Work out the finished part from the listing and answer in its coordinate system (mm). Face numbers are marked on the shaded views. A direction names the side the tool comes from. Give positions to 0.01 mm unless a question says otherwise; leave off trailing zeros. Loops run counter-clockwise (first coordinate to the right, second up) from the corner with the lowest first, then second, coordinate; pieces in that order, holes last. Notation, with made-up numbers: M 83,10 L 114,10 A20 cw 114,25 Z; hole C -2.5,-19 d6. An arc over 180 degrees is marked long. Use a Markdown table: item, result.
```python
from build123d import *

# Parameters (mm, degrees)
BOSS_EXTRUDE1_DEPTH = 1.8
SKETCH2_R           = 3.25
SKETCH2_R_2         = 2.5
BOSS_EXTRUDE3_DEPTH = 0.2
SKETCH4_R           = 3.25
SKETCH4_R_2         = 2
BOSS_EXTRUDE4_DEPTH = 3
CUT_EXTRUDE1_REACH  = 4
SKETCH5_R           = 1.5
CUT_EXTRUDE2_REACH  = 6.8
SKETCH6_R           = 0.5


with BuildPart() as part:
    # Sketch1 → Boss-Extrude1 (new body)
    with BuildSketch(Plane.XY):
        with BuildLine():
            Line((1.525163579, 2.869908719), (15.645, 1.543202838))
            ThreePointArc((15.645, 1.543202838), (17.05, 0), (15.645, -1.543202838))
            Line((15.645, -1.543202838), (1.525163579, -2.869908719))
            ThreePointArc((1.525163579, -2.869908719), (0, -3.25), (-1.525163579, -2.869908719))
            Line((-1.525163579, -2.869908719), (-15.645, -1.543202838))
            ThreePointArc((-15.645, -1.543202838), (-17.05, 0), (-15.645, 1.543202838))
            Line((-15.645, 1.543202838), (-1.525163579, 2.869908719))
            ThreePointArc((-1.525163579, 2.869908719), (0, 3.25), (1.525163579, 2.869908719))
        make_face()
    extrude(amount=BOSS_EXTRUDE1_DEPTH)

    # Sketch2 → Boss-Extrude3 (add)
    with BuildSketch(Plane(origin=(0, 0, 0), x_dir=(-1, 0, 0), z_dir=(0, 0, -1))):
        Circle(SKETCH2_R)
        Circle(SKETCH2_R_2, mode=Mode.SUBTRACT)
    extrude(amount=BOSS_EXTRUDE3_DEPTH)

    # Sketch4 → Boss-Extrude4 (add)
    with BuildSketch(Plane.XY.offset(1.8)):
        Circle(SKETCH4_R)
        Circle(SKETCH4_R_2, mode=Mode.SUBTRACT)
    extrude(amount=BOSS_EXTRUDE4_DEPTH)

    # Sketch5 → Cut-Extrude1 (cut, up to next)
    with BuildSketch(Plane.XY.offset(1.8), mode=Mode.PRIVATE) as cut_extrude1_sk1:
        Circle(SKETCH5_R)
    cut_extrude1_tool1 = extrude(cut_extrude1_sk1.sketch, amount=-CUT_EXTRUDE1_REACH, mode=Mode.PRIVATE) & part.part
    add(cut_extrude1_tool1.solids().sort_by_distance((0, 0, 1.8))[0], mode=Mode.SUBTRACT)

    # Sketch6 → Cut-Extrude2 (cut, up to next)
    with BuildSketch(Plane(origin=(0, 0, 0), x_dir=(-1, 0, 0), z_dir=(0, 0, -1)), mode=Mode.PRIVATE) as cut_extrude2_sk1:
        with Locations((15.5, 0)):
            Circle(SKETCH6_R)
    cut_extrude2_tool1 = extrude(cut_extrude2_sk1.sketch, amount=-CUT_EXTRUDE2_REACH, mode=Mode.PRIVATE) & part.part
    add(cut_extrude2_tool1.solids().sort_by_distance((-15.5, 0, 0))[0], mode=Mode.SUBTRACT)
    # Sketch6 → Cut-Extrude2 (cut, up to next)
    with BuildSketch(Plane(origin=(0, 0, 0), x_dir=(-1, 0, 0), z_dir=(0, 0, -1)), mode=Mode.PRIVATE) as cut_extrude2_sk2:
        with Locations((13.3, 0)):
            Circle(SKETCH6_R)
    cut_extrude2_tool2 = extrude(cut_extrude2_sk2.sketch, amount=-CUT_EXTRUDE2_REACH, mode=Mode.PRIVATE) & part.part
    add(cut_extrude2_tool2.solids().sort_by_distance((-13.3, 0, 0))[0], mode=Mode.SUBTRACT)
    # Sketch6 → Cut-Extrude2 (cut, up to next)
    with BuildSketch(Plane(origin=(0, 0, 0), x_dir=(-1, 0, 0), z_dir=(0, 0, -1)), mode=Mode.PRIVATE) as cut_extrude2_sk3:
        with Locations((11.1, 0)):
            Circle(SKETCH6_R)
    cut_extrude2_tool3 = extrude(cut_extrude2_sk3.sketch, amount=-CUT_EXTRUDE2_REACH, mode=Mode.PRIVATE) & part.part
    add(cut_extrude2_tool3.solids().sort_by_distance((-11.1, 0, 0))[0], mode=Mode.SUBTRACT)
    # Sketch6 → Cut-Extrude2 (cut, up to next)
    with BuildSketch(Plane(origin=(0, 0, 0), x_dir=(-1, 0, 0), z_dir=(0, 0, -1)), mode=Mode.PRIVATE) as cut_extrude2_sk4:
        with Locations((8.9, 0)):
            Circle(SKETCH6_R)
    cut_extrude2_tool4 = extrude(cut_extrude2_sk4.sketch, amount=-CUT_EXTRUDE2_REACH, mode=Mode.PRIVATE) & part.part
    add(cut_extrude2_tool4.solids().sort_by_distance((-8.9, 0, 0))[0], mode=Mode.SUBTRACT)
    # Sketch6 → Cut-Extrude2 (cut, up to next)
    with BuildSketch(Plane(origin=(0, 0, 0), x_dir=(-1, 0, 0), z_dir=(0, 0, -1)), mode=Mode.PRIVATE) as cut_extrude2_sk5:
        with Locations((6.7, 0)):
            Circle(SKETCH6_R)
    cut_extrude2_tool5 = extrude(cut_extrude2_sk5.sketch, amount=-CUT_EXTRUDE2_REACH, mode=Mode.PRIVATE) & part.part
    add(cut_extrude2_tool5.solids().sort_by_distance((-6.7, 0, 0))[0], mode=Mode.SUBTRACT)
    # Sketch6 → Cut-Extrude2 (cut, up to next)
    with BuildSketch(Plane(origin=(0, 0, 0), x_dir=(-1, 0, 0), z_dir=(0, 0, -1)), mode=Mode.PRIVATE) as cut_extrude2_sk6:
        with Locations((4.5, 0)):
            Circle(SKETCH6_R)
    cut_extrude2_tool6 = extrude(cut_extrude2_sk6.sketch, amount=-CUT_EXTRUDE2_REACH, mode=Mode.PRIVATE) & part.part
    add(cut_extrude2_tool6.solids().sort_by_distance((-4.5, 0, 0))[0], mode=Mode.SUBTRACT)
    # Sketch6 → Cut-Extrude2 (cut, up to next)
    with BuildSketch(Plane(origin=(0, 0, 0), x_dir=(-1, 0, 0), z_dir=(0, 0, -1)), mode=Mode.PRIVATE) as cut_extrude2_sk7:
        with Locations((-4.5, 0)):
            Circle(SKETCH6_R)
    cut_extrude2_tool7 = extrude(cut_extrude2_sk7.sketch, amount=-CUT_EXTRUDE2_REACH, mode=Mode.PRIVATE) & part.part
    add(cut_extrude2_tool7.solids().sort_by_distance((4.5, 0, 0))[0], mode=Mode.SUBTRACT)
    # Sketch6 → Cut-Extrude2 (cut, up to next)
    with BuildSketch(Plane(origin=(0, 0, 0), x_dir=(-1, 0, 0), z_dir=(0, 0, -1)), mode=Mode.PRIVATE) as cut_extrude2_sk8:
        with Locations((-6.7, 0)):
            Circle(SKETCH6_R)
    cut_extrude2_tool8 = extrude(cut_extrude2_sk8.sketch, amount=-CUT_EXTRUDE2_REACH, mode=Mode.PRIVATE) & part.part
    add(cut_extrude2_tool8.solids().sort_by_distance((6.7, 0, 0))[0], mode=Mode.SUBTRACT)
    # Sketch6 → Cut-Extrude2 (cut, up to next)
    with BuildSketch(Plane(origin=(0, 0, 0), x_dir=(-1, 0, 0), z_dir=(0, 0, -1)), mode=Mode.PRIVATE) as cut_extrude2_sk9:
        with Locations((-8.9, 0)):
            Circle(SKETCH6_R)
    cut_extrude2_tool9 = extrude(cut_extrude2_sk9.sketch, amount=-CUT_EXTRUDE2_REACH, mode=Mode.PRIVATE) & part.part
    add(cut_extrude2_tool9.solids().sort_by_distance((8.9, 0, 0))[0], mode=Mode.SUBTRACT)
    # Sketch6 → Cut-Extrude2 (cut, up to next)
    with BuildSketch(Plane(origin=(0, 0, 0), x_dir=(-1, 0, 0), z_dir=(0, 0, -1)), mode=Mode.PRIVATE) as cut_extrude2_sk10:
        with Locations((-11.1, 0)):
            Circle(SKETCH6_R)
    cut_extrude2_tool10 = extrude(cut_extrude2_sk10.sketch, amount=-CUT_EXTRUDE2_REACH, mode=Mode.PRIVATE) & part.part
    add(cut_extrude2_tool10.solids().sort_by_distance((11.1, 0, 0))[0], mode=Mode.SUBTRACT)
    # Sketch6 → Cut-Extrude2 (cut, up to next)
    with BuildSketch(Plane(origin=(0, 0, 0), x_dir=(-1, 0, 0), z_dir=(0, 0, -1)), mode=Mode.PRIVATE) as cut_extrude2_sk11:
        with Locations((-13.3, 0)):
            Circle(SKETCH6_R)
    cut_extrude2_tool11 = extrude(cut_extrude2_sk11.sketch, amount=-CUT_EXTRUDE2_REACH, mode=Mode.PRIVATE) & part.part
    add(cut_extrude2_tool11.solids().sort_by_distance((13.3, 0, 0))[0], mode=Mode.SUBTRACT)
    # Sketch6 → Cut-Extrude2 (cut, up to next)
    with BuildSketch(Plane(origin=(0, 0, 0), x_dir=(-1, 0, 0), z_dir=(0, 0, -1)), mode=Mode.PRIVATE) as cut_extrude2_sk12:
        with Locations((-15.5, 0)):
            Circle(SKETCH6_R)
    cut_extrude2_tool12 = extrude(cut_extrude2_sk12.sketch, amount=-CUT_EXTRUDE2_REACH, mode=Mode.PRIVATE) & part.part
    add(cut_extrude2_tool12.solids().sort_by_distance((15.5, 0, 0))[0], mode=Mode.SUBTRACT)


solid = part.part
```
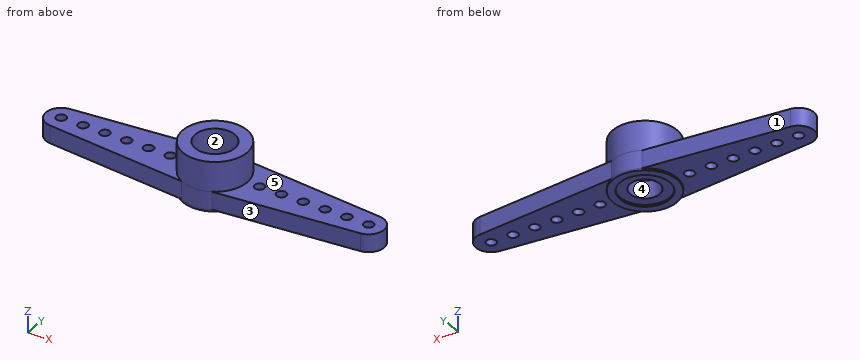
(1) A cutting plane is placed at A-A (z = 1.1). Count the separate pieces of the cut face and the enclosed holes in it, and give its area (3 significant figures).
Entries:
| item | result |
|---|---|
| separate pieces | 1 |
| enclosed holes | 13 |
| area | 134 mm² |
(2) A cutting plane is placed at D-D (x = 6.7). Write down the section's boundary in (y, z).
Entries:
| item | result |
|---|---|
| outline | M -2.38,0 L -0.5,0 L -0.5,1.8 L -2.38,1.8 Z; M 0.5,0 L 2.38,0 L 2.38,1.8 L 0.5,1.8 Z |
(3) A cutting plane is placed at C-C (z = 2.6). Write down the section's boundary in (x, y).
Entries:
| item | result |
|---|---|
| outline | C 0,0 d6.5; hole C 0,0 d4 |
(4) Given P1, Ø3, axis at x = 6, y = 0, coming from the -Z side; P2, Ø1, axis at x = 8, y = 0, coming from the +Z side; P3, Ø2, axis at x = 4, z = 1.5, coming from the -Y side; P4, Ø1.8, axis at x = 0, y = 0, coming from the -Z side, each flat-ended and moving along its own axis, determine where each tip first touches the part or whether it passes through.
Entries:
| item | result |
|---|---|
| P1 | stops at z = 0 |
| P2 | stops at z = 1.8 |
| P3 | stops at y = -2.73 |
| P4 | passes through |
(5) The mould has two halves that part along X. Classify the marked faces 3, 4 and 5: released by +X, released by -X, zero draft, split by the parting line, or undercut.
Entries:
| item | result |
|---|---|
| face 3 | released by +X |
| face 4 | undercut |
| face 5 | zero draft |
(6) A cutting plane is placed at B-B (x = 13.3). Write down the section's boundary in (y, z).
Entries:
| item | result |
|---|---|
| outline | M -1.76,0 L -0.5,0 L -0.5,1.8 L -1.76,1.8 Z; M 0.5,0 L 1.76,0 L 1.76,1.8 L 0.5,1.8 Z |
(7) Which of the six approach directions +Z, -Z, +X, -X, +Y, -Y give full straight-line access (tool end or side, diameter ignored) to the marked faces 1 and 2?
Entries:
| item | result |
|---|---|
| face 1 | +Z, -Z, -X, +Y |
| face 2 | +Z |
(8) Consider probe 1 along Y at (x, z) = (0, 2.85); probe 2 along Z at (x, y) = (9, 2); probe 3 along X at (y, z) = (-1, 2.85). Determine where each line is inside the solid, lowest interval first. Write a range as [from, to].
Entries:
| item | result |
|---|---|
| probe 1 | y = [-3.25, -2], [2, 3.25] |
| probe 2 | z = [0, 1.8] |
| probe 3 | x = [-3.09, -1.73], [1.73, 3.09] |
